Source: CAD feature listing. Evaluate the final solid. Frame: model axes, mm. Give positions to 0.01 mm unless a question says otherwise; leave off trailing zeros. Loops run counter-clockwise (first coordinate to the right, second up) from the corner with the lowest first, then second, coordinate; pieces in that order, holes last. Notation, with made-up numbers: (36.25, -38.75) - (86.25, -38.75) arc R8 cw to (86.25, -26.75) - close; hole circle Ø1 at (66.5, 59). An arc over 180 degrees is marked (long way). Write each question's results on one line, items separated by ' | '. Start each with the question number.
(1) Pull-direction query (X, two-part tool) for faces 1 (the cylindrical face through (204.12, 27.58, -1.48)), 2 (the flat face through (92, 17, 0)); classes: pulls with the +X half, pulls with the -X half, needs draft (parallel to the pull), parting line crosses it, or undercut.
(2) Cut plane A-A on y = 26.75. Return the cut outline in (x, z).
(3) Contact query for a flat-ended pin moving along its axis: pin 1 (3.5 mm diameter, centred on x = -14, y = 6.75, fed in from +Z). Output: stop coordinate, or through.
(4) Material intervals for line 1 along Y through (x, z) = (201.5, -1.65); line 2 along X through (y, z) = (9, -2.65), sorted ascending. Write a range as [from, to].
(5) Cut plane B-B on x = -14. Return the cut outline in (y, z), then the cut area to 3 significant figures.
from build123d import *

# Parameters (mm, degrees)
EXTRUSION_BASE_SKETCH_W      = 231.5
EXTRUSION_BASE_SKETCH_H      = 40
EXTRUSION_BASE_EXTRUDE_DEPTH = 3
M5_MOUNTING_HOLES_D          = 5.5


with BuildPart() as part:
    # Extrusion Base Sketch → Extrusion Base Extrude (new body)
    with BuildSketch(Plane.XY):
        with Locations((93.75, 16.75)):
            Rectangle(EXTRUSION_BASE_SKETCH_W, EXTRUSION_BASE_SKETCH_H)
    extrude(amount=-EXTRUSION_BASE_EXTRUDE_DEPTH)

    # M5 Mounting Holes (through all)
    with Locations(Plane(origin=(0, 0, -3), x_dir=(-1, 0, 0), z_dir=(0, 0, -1))):
        with Locations((-201.5, 26.75), (-201.5, 6.75), (14, 26.75), (14, 6.75)):
            Hole(M5_MOUNTING_HOLES_D / 2)


solid = part.part
Ans:
1) face 1: undercut | face 2: needs draft
2) outline: (-22, -3) - (-16.75, -3) - (-16.75, 0) - (-22, 0) - close; (-11.25, -3) - (198.75, -3) - (198.75, 0) - (-11.25, 0) - close; (204.25, -3) - (209.5, -3) - (209.5, 0) - (204.25, 0) - close
3) pin 1: through
4) line 1: [-3.25, 4], [9.5, 24], [29.5, 36.75] | line 2: [-22, -15.58], [-12.42, 199.92], [203.08, 209.5]
5) outline: (-3.25, -3) - (4, -3) - (4, 0) - (-3.25, 0) - close; (9.5, -3) - (24, -3) - (24, 0) - (9.5, 0) - close; (29.5, -3) - (36.75, -3) - (36.75, 0) - (29.5, 0) - close | area: 87.0 mm^2
